Could you check a few things on this model? Use its own coordinates, in mm. A direction names the side the tool comes from. Give positions to 0.01 mm unless a question says otherwise; leave off trailing zeros. Order: outer loops, then holes, each group sorted by start corner. A loop starts at its lowest first (then second) coordinate and runs counter-clockwise, first axis right, second up. Notation, with made-up numbers: (48, 28.5) -> (105, 28.5) arc R17 ccw to (105, 40.5) -> close; hole circle Ø10 at (38, 51). An arc over 180 degrees is marked (long way). Answer as CSV lines item,"result". Start each with the question number.
(1) I want a section at D-D (x = -0.5). Please give me the cut outline in (y, z) (3 decimals).
(2) On a 3-axis mill with a long thin cutter (end or side, diameter ignored), from which of +Z, -Z, +X, -X, +Y, -Y can I reach the whole of each face in a straight line? I mean faces 1 (the face through (-66.281, 0, 5)), 2 (the face through (69.944, 15.87, 4.829)), 3 (the face through (-45.814, -15.87, 4.829)). Say none if no direction works.
(3) Will these pins go through, and if not, where does the flat tip stop? pin 1 Ø5 at (y, z) = (12, 1.5) entering from +X (3 decimals); pin 2 Ø1.1 at (x, z) = (62.5, 3) entering from -Y; pin 3 Ø0.7 at (x, z) = (-62.5, 4.5) entering from -Y; pin 4 Ø3 at (x, z) = (10, 4.5) entering from +Y.
(4) I need wall thicknesses on L1, parallel to X at y = -6, z = 1.5 (1 decimal); L2, parallel to X at y = 12, z = 8.5; L3, parallel to X at y = 8.5, z = 8.25 (3 decimals). Which ranges of each line are inside material? Lowest first, please.
(5) I want a section at B-B (z = 7). Give the number of separate pieces and of enclosed holes in the cut face, plus the area to 3 significant figures.
(6) We'd pull the mould along Y, two halves only. Please class faces 4 (the face through (1.02, -35.43, 4.7)), 5 (the face through (49.535, 15.969, 4.829)), 6 (the face through (-59.565, -8.62, 4.829)), 7 (the face through (0, -19, 9.525)): released by +Y, released by -Y, zero draft, split by the parting line, or undercut.
(7) I want a section at C-C (y = -8). Please give me the cut outline in (x, z) (3 decimals).
(8) I want a section at A-A (y = -1). Please give me the cut outline in (x, z) (1 decimal).
Autodesk Inventor part; units mm, degrees
sketch "Sketch1" plane through (0, 0, 0) normal (0, 0, 1) x (1, 0, 0)
  line L0 (-100.457, 0) -> (100.457, 0) construction
  line L1 (0, 116.967) -> (0, -60.833) construction
  circle A0 centre (-62.4459, 0) radius 3.8354 construction
  circle A1 centre (62.4459, 0) radius 3.8354 construction
  line L2 (-62.4459, 0) -> (62.4459, 0) construction
  line L3 (-71.755, 17.78) -> (71.755, 17.78)
  line L4 (71.755, 17.78) -> (71.755, -13.2195)
  line L5 (-71.755, -13.2195) -> (-71.755, 17.78)
  circle A2 centre (-64.3509, 0) radius 3.8354 construction
  circle A3 centre (-60.5409, 0) radius 3.8354 construction
  line L6 (-64.3559, 3.8354) -> (-60.5409, 3.8354) construction
  line L7 (-64.3763, -3.8353) -> (-60.541, -3.8354) construction
  circle A4 centre (62.4459, 0) radius 3.8354 construction
  arc A5 (-71.755, -13.2195) -> (71.755, -13.2195) centre (0, 91.567) ccw
  line L8 (66.2813, -9.525) -> (58.6105, -9.525)
  line L9 (58.6105, -9.525) -> (58.6105, 9.525)
  line L10 (58.6105, 9.525) -> (66.2813, 9.525)
  line L11 (66.2813, 9.525) -> (66.2813, -9.525)
  line L12 (66.2813, -9.525) -> (58.6105, 9.525) construction
  line L13 (58.6105, -9.525) -> (66.2813, 9.525) construction
  line L14 (-58.6105, -9.525) -> (-66.2813, -9.525)
  line L15 (-66.2813, -9.525) -> (-66.2813, 9.525)
  line L16 (-66.2813, 9.525) -> (-58.6105, 9.525)
  line L17 (-58.6105, 9.525) -> (-58.6105, -9.525)
  line L18 (-58.6105, -9.525) -> (-66.2813, 9.525) construction
  line L19 (-66.2813, -9.525) -> (-58.6105, 9.525) construction
  point P0 (0, 0)
  point P1 (0, 0)
  point P2 (0, 17.78)
  dimension "d0" = 7.6708
  dimension "d1" = 124.8918
  dimension "d2" = 143.51
  dimension "d3" = 17.78
  dimension "d16" = 7.6708
  dimension "d17" = 1.905
  dimension "d18" = 1.905
  dimension "d33" = 127
  dimension "d34" = 19.05
  dimension "d35" = 19.05
  dimension "d36" = 7.6708
  dimension "d37" = 35.433
ref_plane "Work Plane1" through (0, -74.9046, 0) normal (0, 1, 0) x (-1, 0, 0)
ref_plane "Work Plane2" through (0, -1.905, 0) normal (0, 1, 0) x (-1, 0, 0)
extrude "Extrusion1" add sketch "Sketch1" along normal blind 9.525 contours L3 L4 A5 L5 | L8 L9 L10 L11 | L14 L15 L16 L17
extrude "Extrusion3" cut sketch "Sketch1" along normal blind 9.525 contours L8 L9 L10 L11 | L14 L15 L16 L17
sketch "Sketch4" plane through (0, 0, 0) normal (0, 0, 1) x (1, 0, 0)
  line L0 (-71.755, 17.78) -> (71.755, 17.78)
  line L1 (-47.625, 17.78) -> (47.625, 17.78)
  line L2 (47.625, 17.78) -> (47.625, -17.78)
  line L3 (47.625, -17.78) -> (-47.625, -17.78)
  line L4 (-47.625, -17.78) -> (-47.625, 17.78)
  line L5 (0, -17.78) -> (0, 17.78) construction
  point P0 (0, 0)
  dimension "d21" = 35.56
  dimension "d22" = 95.25
  dimension "d23" = 0
extrude "Extrusion4" cut sketch "Sketch4" along normal up to next
fillet "Fillet2" radius 6.35 8 edges at (-47.625, -17.78, 4.7625) (-47.625, 17.78, 4.7625) (-71.755, 17.78, 4.7625) (47.625, -17.78, 4.7625) (47.625, 17.78, 4.7625) (71.755, 17.78, 4.7625) (71.755, -13.2195, 4.7625) (-71.755, -13.2195, 4.7625)
fillet "Fillet4" radius 3.175 8 edges at (-66.2813, 9.525, 4.7625) (-58.6105, 9.525, 4.7625) (-58.6105, -9.525, 4.7625) (-66.2813, -9.525, 4.7625) (58.6105, 9.525, 4.7625) (66.2813, 9.525, 4.7625) (66.2813, -9.525, 4.7625) (58.6105, -9.525, 4.7625)
sketch "Sketch5" plane through (0, 0, 0) normal (0, 0, 1) x (1, 0, 0)
  line L0 (-100.457, -1.905) -> (100.457, -1.905)
  line L1 (-62.4459, 0) -> (-62.4459, -1.905)
  line L2 (62.4459, 0) -> (62.4459, -1.905)
  point P0 (0, 0)
properties part number "J005684"
Final values:
1,outline,"(-35.432, 0) -> (-17.78, 0) -> (-17.78, 9.525) -> (-35.432, 9.525) -> close"
2,face 1,"+Z, -Z"
2,face 2,"+Z, -Z, +X, +Y"
2,face 3,"+Z, -Z, +Y"
3,pin 1,"x = 71.755"
3,pin 2,"y = -19.3"
3,pin 3,"y = -19.19"
3,pin 4,"y = -17.78"
4,L1,"-71.8 to -66.3, -58.6 to -47.6, 47.6 to 58.6, 66.3 to 71.8"
4,L2,"-71.73 to -47.65, 47.65 to 71.73"
4,L3,"-71.755 to -65.443, -59.449 to -47.625, 47.625 to 59.449, 65.443 to 71.755"
5,separate pieces,"1"
5,enclosed holes,"2"
5,area,"2,930 mm²"
6,face 4,"released by -Y"
6,face 5,"released by +Y"
6,face 6,"undercut"
6,face 7,"zero draft"
7,outline,"(-71.755, 0) -> (-65.819, 0) -> (-65.819, 9.525) -> (-71.755, 9.525) -> close; (-59.073, 0) -> (-47.625, 0) -> (-47.625, 9.525) -> (-59.073, 9.525) -> close; (47.625, 0) -> (59.073, 0) -> (59.073, 9.525) -> (47.625, 9.525) -> close; (65.819, 0) -> (71.755, 0) -> (71.755, 9.525) -> (65.819, 9.525) -> close"
8,outline,"(-71.8, 0) -> (-66.3, 0) -> (-66.3, 9.5) -> (-71.8, 9.5) -> close; (-58.6, 0) -> (-47.6, 0) -> (-47.6, 9.5) -> (-58.6, 9.5) -> close; (47.6, 0) -> (58.6, 0) -> (58.6, 9.5) -> (47.6, 9.5) -> close; (66.3, 0) -> (71.8, 0) -> (71.8, 9.5) -> (66.3, 9.5) -> close"
